Check sheet for the drawn part. Datum: minimum x, y, z corner. Units: mm. Give positions to 0.01 mm unless a question says otherwise; leave off trailing zeros. Loops run counter-clockwise (first coordinate to the right, second up) from the corner with the lowest first, then second, coordinate; pieces in that order, holes last.
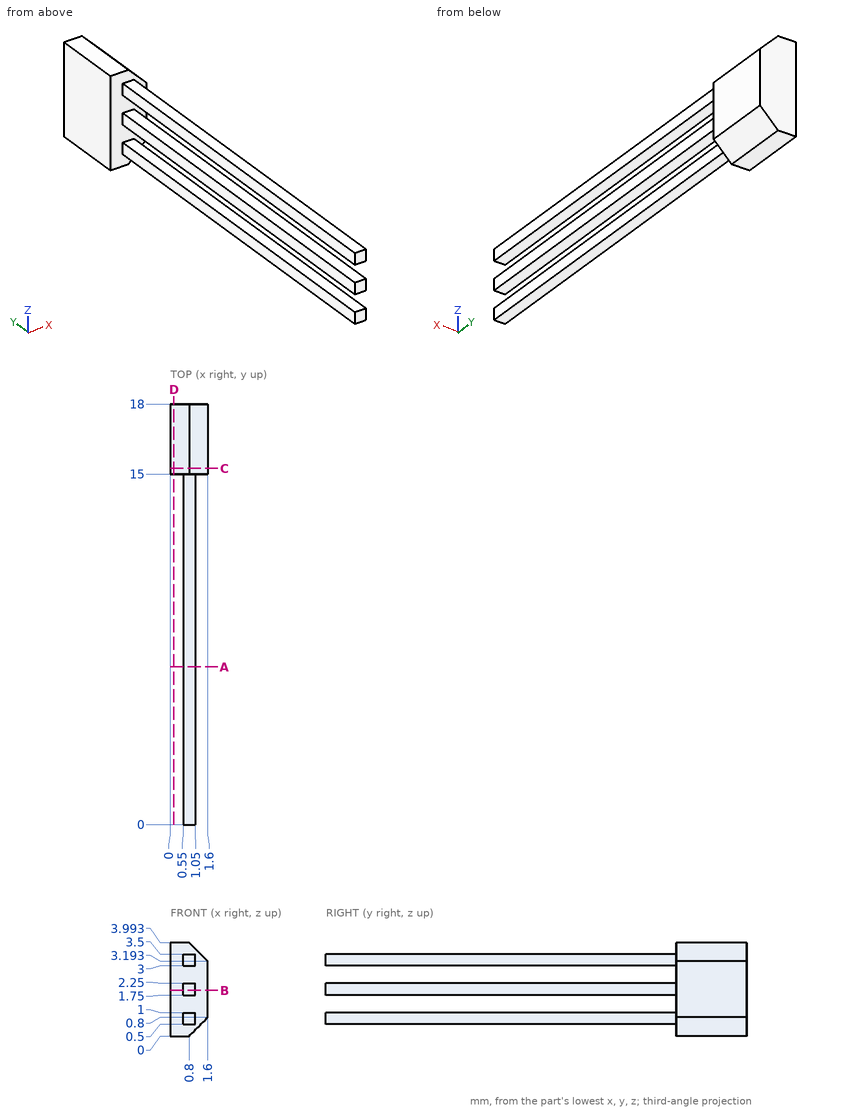
(1) Section check C-C on y = 15.25. Record the boundary of the cut face in (x, z).
(2) Gauge pin test, flat end, axial feed: pin 1 Ø1.5 at (y, z) = (5.5, 2) entering from -X. Record the tip position at first contact, or that the pin passes through.
(3) Material ranges on line 1 (Z direction, x = 0.8, y = 11); line 2 (Y direction, x = 0.15, z = 2.15); line 3 (X direction, y = 1, z = 3.45), recorded low to high.
(4) Section check A-A on y = 6.75. Record the boundary of the cut face in (x, z).
(5) Section check B-B on z = 1.95. Record the boundary of the cut face in (x, y).
(6) Section check D-D on x = 0.15. Record the boundary of the cut face in (y, z).
Computed values:
1. outline: (0, 0) - (0.8, 0) - (1.6, 0.8) - (1.6, 3.19) - (0.8, 3.99) - (0, 3.99) - close
2. pin 1: stops at x = 0.55
3. line 1: z = 0.5 to 1, 1.75 to 2.25, 3 to 3.5
3. line 2: y = 15 to 18
3. line 3: x = 0.55 to 1.05
4. outline: (0.55, 0.5) - (1.05, 0.5) - (1.05, 1) - (0.55, 1) - close; (0.55, 1.75) - (1.05, 1.75) - (1.05, 2.25) - (0.55, 2.25) - close; (0.55, 3) - (1.05, 3) - (1.05, 3.5) - (0.55, 3.5) - close
5. outline: (0, 15) - (0.55, 15) - (0.55, 0) - (1.05, 0) - (1.05, 15) - (1.6, 15) - (1.6, 18) - (0, 18) - close
6. outline: (15, 0) - (18, 0) - (18, 3.99) - (15, 3.99) - close
